```python
from build123d import *

# Parameters (mm, degrees)
PAD013_DEPTH    = 10.5
SKETCH042_R     = 2
POCKET028_DEPTH = 7
CHAMFER019_SIZE = 1
CHAMFER020_SIZE = 2.5


with BuildPart() as part:
    # Sketch041 → Pad013 (new body)
    with BuildSketch(Plane.XY):
        Polygon((26.5, 18.125), (26.5, -18.125), (15, -18.125), (10, -12.5), (0, -12.5), (0, 12.5), (10, 12.5), (15, 18.125), align=None)
    extrude(amount=PAD013_DEPTH)

    # Sketch042 (on Face3 of Pad013) → Pocket028 (cut)
    with BuildSketch(Plane.YZ.offset(26.5)):
        with Locations((-13.625, 3.7)):
            Circle(SKETCH042_R)
        with Locations((13.625, 3.7)):
            Circle(SKETCH042_R)
    extrude(amount=-POCKET028_DEPTH, mode=Mode.SUBTRACT)

    # Chamfer019
    chamfer019_edges = [part.edges().sort_by_distance(p)[0] for p in [
        (20.75, -18.125, 10.5),
        (12.5, -15.3125, 10.5),
        (5, -12.5, 10.5),
        (5, 12.5, 10.5),
        (12.5, 15.3125, 10.5),
        (20.75, 18.125, 10.5),
    ]]
    chamfer(chamfer019_edges, length=CHAMFER019_SIZE)

    # Chamfer020
    chamfer020_edges = [part.edges().sort_by_distance(p)[0] for p in [
        (5, -12.5, 0),
        (12.5, -15.3125, 0),
        (20.75, -18.125, 0),
        (5, 12.5, 0),
        (12.5, 15.3125, 0),
        (20.75, 18.125, 0),
    ]]
    chamfer(chamfer020_edges, length=CHAMFER020_SIZE)


with BuildPart() as part_1:
    # Body004007 placement: moved
    add(part.part.moved(Location((25.3, -7, 6.5))))


solid = part_1.part
```
Can you work these out from the model? Positions are in its coordinate system, mm. A direction names the side the tool comes from. Round coordinates to 2 decimals unless told otherwise and drop trailing zeros. Loops run counter-clockwise (first coordinate to the right, second up) from the corner with the lowest first, then second, coordinate; pieces in that order, holes last. Notation, with made-up numbers: M 9,78 L 67,78 A17 ccw 67,101 Z; hole C 26,15 d2. An arc over 180 degrees is marked long. Answer as a JSON object with one key per item and string values. Group by question number.
Q1. Imagine slicing it at D-D, the plane y = 9. Please give me the cut outline in (x, z) (3 decimals).
Q2. We'd pull the mould along Y, two halves only. Please class faces 5 (the flat face through (30.5, 5, 16.5)), 6 (the flat face through (39, -7, 17)), 7 (the flat face through (44.8, -21, 10)): +Y half, -Y half, draft (parallel to the pull), parting line (faces both ways), or undercut.
Q3. Imagine slicing it at B-B, the plane z = 10.2. Please give me the cut outline in (x, y) (3 decimals).
Q4. Will these pins go through, and if not, where does the flat tip stop? pin 1 (4.5 mm diameter, centred on y = 6.625, z = 10.2, fed in from +X); pin 2 (3.5 mm diameter, centred on x = 30.5, z = 11, fed in from -Y).
Q5. Please list where these lines run through material, in increasing order: L1, parallel to Y at x = 27, z = 11; L2, parallel to Y at x = 40.5, z = 16.5; L3, parallel to X at y = 7, z = 8.75.
Q6. Imagine slicing it at A-A, the plane x = 45.5. Please give me the cut outline in (y, z) (3 decimals), then the cut area to 3 significant figures.
Q7. Imagine slicing it at C-C, the plane x = 28.75. Please give me the cut outline in (y, z), then the cut area to 3 significant figures.
Q8. On a 3-axis mill with a long thin cutter (end or side, diameter ignored), from which of +Z, -Z, +X, -X, +Y, -Y can I reach the whole of each face in a straight line? I mean faces 1 (the flat face through (38.308, 7.029, 7.768)), 2 (the flat face through (30.9, -18.3, 7.8)), 3 (the flat face through (44.8, 7, 10)), 4 (the flat face through (30, 5.5, 12)). Say none if no direction works.
Findings:
{
 "1": {"outline": "M 38.411,9 L 41.254,6.875 L 51.8,6.875 L 51.8,17 L 39.749,17 L 38.411,16 Z"},
 "2": {"face 5": "+Y half", "face 6": "draft", "face 7": "undercut"},
 "3": {"outline": "M 25.3,-19.5 L 35.3,-19.5 L 40.3,-25.125 L 51.8,-25.125 L 51.8,-22.625 L 44.8,-22.625 L 44.8,-18.625 L 51.8,-18.625 L 51.8,4.625 L 44.8,4.625 L 44.8,8.625 L 51.8,8.625 L 51.8,11.125 L 40.3,11.125 L 35.3,5.5 L 25.3,5.5 Z"},
 "4": {"pin 1": "stops at x = 51.8", "pin 2": "stops at y = -19.5"},
 "5": {"L1": "y = -19.5 to 5.5", "L2": "y = -24.6 to 10.6", "L3": "x = 36.97 to 44.8"},
 "6": {"outline": "M -25.125,9 L -22.625,6.5 L 8.625,6.5 L 11.125,9 L 11.125,16 L 10.125,17 L -24.125,17 L -25.125,16 Z; hole C -20.625,10.2 d4; hole C 6.625,10.2 d4", "area": "348 mm2"},
 "7": {"outline": "M -19.5,9 L -17,6.5 L 3,6.5 L 5.5,9 L 5.5,16 L 4.5,17 L -18.5,17 L -19.5,16 Z", "area": "255 mm2"},
 "8": {"face 1": "-Z, -X, +Y", "face 2": "-Z, -X, -Y", "face 3": "+X", "face 4": "+Z, -Z, -X, +Y"}
}
